Model file for the job. Use its own axes, mm. A direction names the side the tool comes from. Give positions to 0.01 mm unless a question says otherwise; leave off trailing zeros. Order: outer loops, then holes, each group sorted by start corner. A loop starts at its lowest first (then second) coordinate and runs counter-clockwise, first axis right, second up. Notation, with made-up numbers: (40.5, 80.25) - (55.5, 80.25) arc R14 ccw to (55.5, 96.25) - close; hole circle Ø7 at (13.5, 78). An arc over 180 degrees is marked (long way). Use CSV: the item, a comma, the result in double quotes. Start each with the question number.
(1) Band-saw the part on B-B, the plane x = 0. Give the cut face in (y, z) (1 decimal), then the cut area to 3 significant figures.
(2) Band-saw the part on C-C, the plane y = -1.5. Count the separate pieces of the cut face and the enclosed holes in it, then the cut area to 3 significant figures.
(3) Pull direction Y, two halves, no side cores. Call faces 5 (the flat face through (11, -2, 4.445)), 6 (the cylindrical face through (5.3, 1.67, 25.65)), 7 (the flat face through (0, 3.437, 42)), 8 (the flat face through (-9.03, -7.7, 12.04)): +Y half, -Y half, draft (parallel to the pull), parting line (faces both ways), or undercut.
(4) Tool access for faces 1 (the flat face through (-2.157, 11.673, 12.036)), 2 (the cylindrical face through (2.7, -4.86, 8.01)), 3 (the flat face through (0, -3.437, 42)), 4 (the cylindrical face through (5.557, 0.087, 12.036)): list every direction of +Z, -Z, +X, -X, +Y, -Y with a clear straight run to the whole face (end or side of a thin tool).
(5) Probe L1, parallel to Y at x = 0, z = 11; L2, parallel to Y at x = 4.75, z = 12.5; L3, parallel to X at y = -1.25, z = 36. List the from-to ranges inside material, lowest first.
(6) Band-saw the part on A-A, the plane z = 6. Give the cut face in (x, y) (1 decimal).
(7) Band-saw the part on D-D, the plane z = 21.5. Give the cut face in (x, y).
(8) Drop flat-ended pins along their axis: pin 1 Ø6 at (x, y) = (3.5, 10) entering from +Z; pin 2 Ø0.8 at (x, z) = (0, 41.5) entering from -Y; pin 3 Ø4.5 at (x, y) = (-3.5, 9) entering from +Z (3 decimals). Give the stop position or say it passes through.
from build123d import *

# Parameters (mm, degrees)
F0_R      = 13.49375
F0_R_2    = 2.15265
F1_DEPTH  = 19.4183
F5_DEPTH  = 14.9733
F7_DEPTH  = 16.2433
F8_R      = 5.55625
F8_R_2    = 2.15265
F9_DEPTH  = 12.6492
F10_R     = 3.96875
F10_R_2   = 2.15265
F11_DEPTH = 8.89
F12_R     = 2.15265
F13_DEPTH = 1.5875


with BuildPart() as f1:
    # F0 (on Top) → F1 (new body)
    with BuildSketch(Plane.XY):
        Circle(F0_R)
        with Locations((-4.7625, -8.248892)):
            Circle(F0_R_2, mode=Mode.SUBTRACT)
        with Locations((4.7625, -8.248892)):
            Circle(F0_R_2, mode=Mode.SUBTRACT)
        with Locations((-9.525, 0)):
            Circle(F0_R_2, mode=Mode.SUBTRACT)
        with Locations((-4.7625, 8.248892)):
            Circle(F0_R_2, mode=Mode.SUBTRACT)
        Circle(F0_R_2, mode=Mode.SUBTRACT)
        with Locations((9.525, 0)):
            Circle(F0_R_2, mode=Mode.SUBTRACT)
        with Locations((4.7625, 8.248892)):
            Circle(F0_R_2, mode=Mode.SUBTRACT)
    extrude(amount=F1_DEPTH)

    # F4 (on face) → F5 (cut, through all)
    with BuildSketch(Plane.XY.offset(19.4183)):
        with BuildLine():
            Line((-3.309837, 13.670305), (-10.183913, 9.701555))
            Line((-10.183913, 9.701555), (-8.199538, 6.264517))
            ThreePointArc((-8.199538, 6.264517), (-2.778125, 4.811854), (-1.325462, 10.233267))
            Line((-1.325462, 10.233267), (-3.309837, 13.670305))
        make_face()
        with BuildLine():
            Line((13.49375, 3.96875), (9.525, 3.96875))
            ThreePointArc((9.525, 3.96875), (5.55625, 0), (9.525, -3.96875))
            Line((9.525, -3.96875), (13.49375, -3.96875))
            Line((13.49375, -3.96875), (13.49375, 3.96875))
        make_face()
        with BuildLine():
            Line((-8.199538, -6.264517), (-10.183913, -9.701555))
            Line((-10.183913, -9.701555), (-3.309837, -13.670305))
            Line((-3.309837, -13.670305), (-1.325462, -10.233267))
            ThreePointArc((-1.325462, -10.233267), (-2.778125, -4.811854), (-8.199538, -6.264517))
        make_face()
    extrude(amount=-F5_DEPTH, mode=Mode.SUBTRACT)

    # F6 (on face) → F7 (cut, through all)
    with BuildSketch(Plane(origin=(0, 0, 0), x_dir=(1, 0, 0), z_dir=(0, 0, -1))):
        with BuildLine():
            Line((1.325462, -10.233267), (3.309837, -13.670305))
            Line((3.309837, -13.670305), (10.183913, -9.701555))
            Line((10.183913, -9.701555), (8.199538, -6.264517))
            ThreePointArc((8.199538, -6.264517), (2.778125, -4.811854), (1.325462, -10.233267))
        make_face()
        with BuildLine():
            Line((10.183913, 9.701555), (3.309837, 13.670305))
            Line((3.309837, 13.670305), (1.325462, 10.233267))
            ThreePointArc((1.325462, 10.233267), (2.778125, 4.811854), (8.199538, 6.264517))
            Line((8.199538, 6.264517), (10.183913, 9.701555))
        make_face()
        with BuildLine():
            Line((-9.525, 3.96875), (-13.49375, 3.96875))
            Line((-13.49375, 3.96875), (-13.49375, -3.96875))
            Line((-13.49375, -3.96875), (-9.525, -3.96875))
            ThreePointArc((-9.525, -3.96875), (-5.55625, 0), (-9.525, 3.96875))
        make_face()
    extrude(amount=-F7_DEPTH, mode=Mode.SUBTRACT)

    # F8 (on face) → F9 (join)
    with BuildSketch(Plane.XY.offset(19.4183)):
        Circle(F8_R)
        Circle(F8_R_2, mode=Mode.SUBTRACT)
    extrude(amount=F9_DEPTH)

    # F10 (on face) → F11 (join)
    with BuildSketch(Plane.XY.offset(32.0675)):
        Circle(F10_R)
        Circle(F10_R_2, mode=Mode.SUBTRACT)
    extrude(amount=F11_DEPTH)

    # F12 (on face) → F13 (join)
    with BuildSketch(Plane.XY.offset(40.9575)):
        Polygon((1.984375, 3.437038), (-1.984375, 3.437038), (-3.96875, 0), (-1.984375, -3.437038), (1.984375, -3.437038), (3.96875, 0), align=None)
        Circle(F12_R, mode=Mode.SUBTRACT)
    extrude(amount=F13_DEPTH)


solid = f1.part
Answer block:
1,outline,"(-13.5, 0) - (-2.2, 0) - (-2.2, 42.5) - (-3.4, 42.5) - (-3.4, 41) - (-4, 41) - (-4, 32.1) - (-5.6, 32.1) - (-5.6, 19.4) - (-13.5, 19.4) - close; (2.2, 0) - (13.5, 0) - (13.5, 19.4) - (5.6, 19.4) - (5.6, 32.1) - (4, 32.1) - (4, 41) - (3.4, 41) - (3.4, 42.5) - (2.2, 42.5) - close"
1,area,"563 mm2"
2,separate pieces,"4"
2,enclosed holes,"0"
2,area,"340 mm2"
3,face 5,"undercut"
3,face 6,"parting line"
3,face 7,"+Y half"
3,face 8,"-Y half"
4,face 1,"+Z, -X"
4,face 2,"-Z"
4,face 3,"+Z, +X, -X, -Y"
4,face 4,"+Z, +X"
5,L1,"y = -13.49 to -2.15, 2.15 to 13.49"
5,L2,"y = -4.28 to 4.28"
5,L3,"x = -3.77 to -1.75, 1.75 to 3.77"
6,outline,"(-12.9, -4) arc R13.5 ccw to (-9.9, -9.2) - (-8.2, -6.3) arc R4 cw to (-1.3, -10.2) - (-3, -13.2) arc R13.5 ccw to (3, -13.2) - (1.3, -10.2) arc R4 cw to (8.2, -6.3) - (9.9, -9.2) arc R13.5 ccw to (12.9, -4) - (9.5, -4) arc R4 cw to (9.5, 4) - (12.9, 4) arc R13.5 ccw to (9.9, 9.2) - (8.2, 6.3) arc R4 cw to (1.3, 10.2) - (3, 13.2) arc R13.5 ccw to (-3, 13.2) - (-1.3, 10.2) arc R4 cw to (-8.2, 6.3) - (-9.9, 9.2) arc R13.5 ccw to (-12.9, 4) - (-9.5, 4) arc R4 cw to (-9.5, -4) - close; hole circle Ø4.3 at (0, 0)"
7,outline,"circle Ø11.11 at (0, 0); hole circle Ø4.31 at (0, 0)"
8,pin 1,"stops at z = 19.42"
8,pin 2,"stops at y = -3.44"
8,pin 3,"stops at z = 4.445"
